Build history of the part. All positions in model axes, mm. A direction names the side the tool comes from. Coordinates: 2 decimals unless noted, no trailing zeros. Order: outer loops, then holes, each group sorted by start corner. A loop starts at its lowest first (then second) coordinate and runs counter-clockwise, first axis right, second up. Notation, with made-up numbers: (19, 85) - (37, 85) arc R21 cw to (37, 114) - close; hole circle Ø3 at (88.25, 76.25). An arc over 180 degrees is marked (long way). Write each question's results on one line, items separated by ' | '.
from build123d import *

# Parameters (mm, degrees)
SKETCH1_W           = 40
SKETCH1_H           = 30
SKETCH1_R           = 1.5
BOSS_EXTRUDE1_DEPTH = 3
SKETCH2_W           = 40
SKETCH2_H           = 3
BOSS_EXTRUDE2_DEPTH = 50
FILLET1_R           = 5
SKETCH3_R           = 8
CUT_EXTRUDE1_DEPTH  = 3


with BuildPart() as part:
    # Sketch1 → Boss-Extrude1 (new body)
    with BuildSketch(Plane.XY):
        Rectangle(SKETCH1_W, SKETCH1_H)
        with Locations((-10, 8)):
            Circle(SKETCH1_R, mode=Mode.SUBTRACT)
        with Locations((10, 8)):
            Circle(SKETCH1_R, mode=Mode.SUBTRACT)
        with Locations((-10, -12)):
            Circle(SKETCH1_R, mode=Mode.SUBTRACT)
        with Locations((10, -12)):
            Circle(SKETCH1_R, mode=Mode.SUBTRACT)
    extrude(amount=BOSS_EXTRUDE1_DEPTH)

    # Sketch2 → Boss-Extrude2 (add)
    with BuildSketch(Plane.XY.offset(3)):
        with Locations((0, 13.5)):
            Rectangle(SKETCH2_W, SKETCH2_H)
    extrude(amount=BOSS_EXTRUDE2_DEPTH)

    # Fillet1
    fillet1_edges = [part.edges().sort_by_distance(p)[0] for p in [
        (-20, 13.5, 53),
        (20, 13.5, 53),
    ]]
    fillet(fillet1_edges, radius=FILLET1_R)

    # Sketch3 → Cut-Extrude1 (cut)
    with BuildSketch(Plane(origin=(0, 15, 0), x_dir=(1, 0, 0), z_dir=(0, 1, 0))):
        with Locations(Location((0, -28.681080483, 0), (0, 0, 270))):
            Circle(SKETCH3_R)
    extrude(amount=-CUT_EXTRUDE1_DEPTH, mode=Mode.SUBTRACT)


solid = part.part
1. Band-saw the part on D-D on z = 30. Give the cut face in (x, y), then the cut area to 3 significant figures.
Solved:
outline: (-20, 12) - (-7.89, 12) - (-7.89, 15) - (-20, 15) - close; (7.89, 12) - (20, 12) - (20, 15) - (7.89, 15) - close | area: 72.7 mm2
2. Probe line 1 (Y direction, x = 10, z = 2); line 2 (Y direction, x = 11, z = 29.5); line 3 (Z direction, x = -2, y = -13.5). List the from-to ranges inside material, lowest first.
Solved:
line 1: y = -15 to -13.5, -10.5 to 6.5, 9.5 to 15 | line 2: y = 12 to 15 | line 3: z = 0 to 3
3. Band-saw the part on A-A on x = 10. Give the cut face in (y, z).
Solved:
outline: (-15, 0) - (-13.5, 0) - (-13.5, 3) - (-15, 3) - close; (-10.5, 0) - (6.5, 0) - (6.5, 3) - (-10.5, 3) - close; (9.5, 0) - (15, 0) - (15, 53) - (12, 53) - (12, 3) - (9.5, 3) - close
4. Two-plate mould, pull along X, no slides. Class faces 3 (the face through (19, 14, 51)), 4 (the face through (-7.1, 13.52, 32.37)), 5 (the face through (-11.2, 7.1, 1.5)), 6 (the face through (-20, 12.2, 15)): +X half, -X half, draft (parallel to the pull), parting line (faces both ways), or undercut.
Solved:
face 3: +X half | face 4: undercut | face 5: undercut | face 6: -X half
5. Drop flat-ended pins along their axis: pin 1 Ø4 at (x, y) = (-10, -12) entering from +Z; pin 2 Ø2 at (x, z) = (-9, 37) entering from -Y. Give the stop position or say it passes through.
Solved:
pin 1: stops at z = 3 | pin 2: stops at y = 12
6. Band-saw the part on C-C on x = 0. Give the cut face in (y, z).
Solved:
outline: (-15, 0) - (15, 0) - (15, 20.68) - (12, 20.68) - (12, 3) - (-15, 3) - close; (12, 36.68) - (15, 36.68) - (15, 53) - (12, 53) - close
7. Band-saw the part on B-B on y = -12. Give the cut face in (x, z).
Solved:
outline: (-20, 0) - (-11.5, 0) - (-11.5, 3) - (-20, 3) - close; (-8.5, 0) - (8.5, 0) - (8.5, 3) - (-8.5, 3) - close; (11.5, 0) - (20, 0) - (20, 3) - (11.5, 3) - close
8. Tool access for faces 1 (the face through (0, -15, 1)), 2 (the face through (-5, 12, 22)): list every direction of +Z, -Z, +X, -X, +Y, -Y with a clear straight run to the whole face (end or side of a thin tool).
Solved:
face 1: +Z, -Z, +X, -X, -Y | face 2: +Z, +X, -X, -Y
